Geometry check sheet. Reference: drawing and pictorial views, mm from the part's lowest x, y, z. Coordinates: 2 decimals unless noted, no trailing zeros. Write each loop counter-clockwise with the first axis right and the second up, starting at its lowest first coordinate (ties: lowest second). Pieces come first, ordered by that corner, then holes. Notation, with made-up numbers: (38.25, -16) - (56.25, -16) arc R28 ccw to (56.25, 14) - close; hole circle Ø6 at (-4, -13.75). An arc over 180 degrees is marked (long way). Use one line per item in the form item = value. Start each with the question number.
(1) Gauge pin test, flat ends, axial feed: pin 1 Ø2 at (y, z) = (2, 67.5) entering from -X; pin 2 Ø3 at (x, z) = (161, 89.5) entering from +Y. Record the tip position at first contact, or that the pin passes through.
(2) Sectioned sample at A-A (x = 170). Record the cut outline in (y, z).
(3) Sectioned sample at C-C (z = 30). Record the cut outline in (x, y).
(4) Material ranges on line 1 (X direction, y = 3.45, z = 30); line 2 (Z direction, x = 30, y = 3.95); line 3 (Y direction, x = 181.5, z = 56), recorded low to high. Write a range as [from, to].
(5) Sectioned sample at B-B (y = 11.25). Record the cut outline in (x, z).
(6) Sectioned sample at D-D (x = 67.5). Record the cut outline in (y, z), and give its area (3 significant figures).
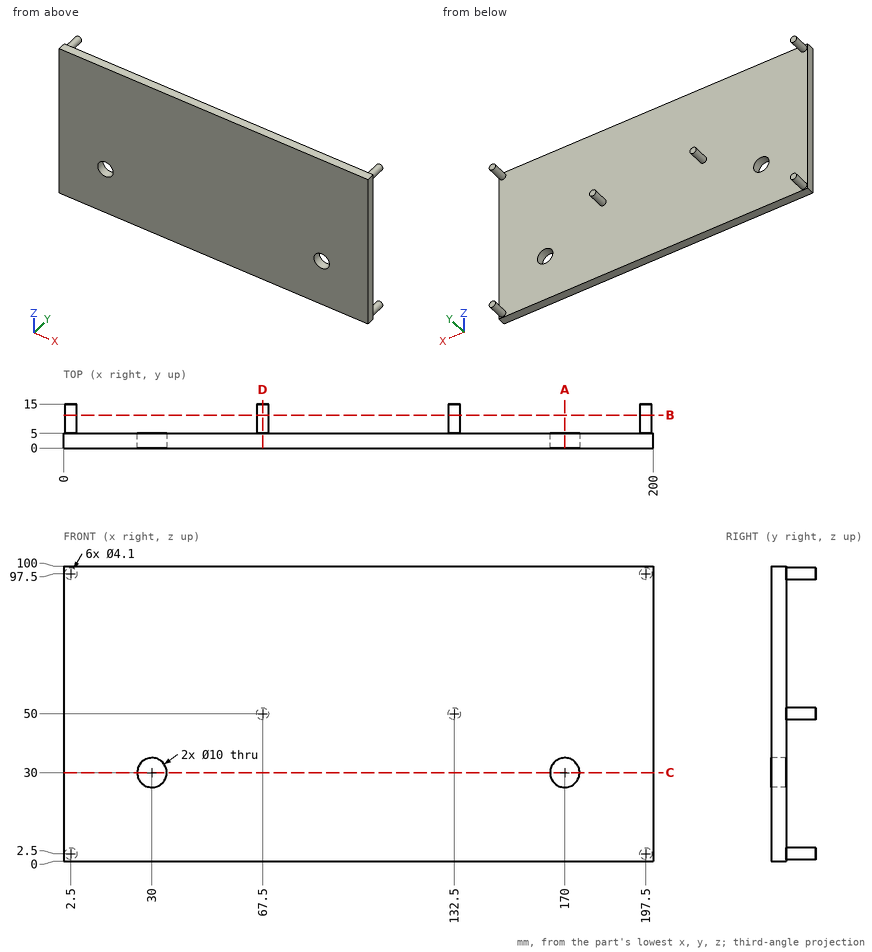
Answers below:
q1.pin_1 = 0
q1.pin_2 = 5
q2.outline = (0, 0) - (5, 0) - (5, 25) - (0, 25) - close; (0, 35) - (5, 35) - (5, 100) - (0, 100) - close
q3.outline = (0, 0) - (25, 0) - (25, 5) - (0, 5) - close; (35, 0) - (165, 0) - (165, 5) - (35, 5) - close; (175, 0) - (200, 0) - (200, 5) - (175, 5) - close
q4.line_1 = [0, 25], [35, 165], [175, 200]
q4.line_2 = [0, 25], [35, 100]
q4.line_3 = [0, 5]
q5.outline = circle Ø4.1 at (2.5, 2.5); circle Ø4.1 at (2.5, 97.5); circle Ø4.1 at (67.5, 50); circle Ø4.1 at (132.5, 50); circle Ø4.1 at (197.5, 2.5); circle Ø4.1 at (197.5, 97.5)
q6.outline = (0, 0) - (5, 0) - (5, 47.95) - (15, 47.95) - (15, 52.05) - (5, 52.05) - (5, 100) - (0, 100) - close
q6.area = 541 mm2
